from build123d import *

# Parameters (mm, degrees)
SZKIC1_W                    = 300
SZKIC1_H                    = 200
DODANIE_WYCI_GNI_CIE1_DEPTH = 2
WYTNIJ_WYCI_GNI_CIE1_REACH  = 182.289
SZKIC2_R                    = 1.5
WYTNIJ_WYCI_GNI_CIE2_DEPTH  = 2


with BuildPart() as part:
    # Szkic1 → Dodanie-wyciągnięcie1 (new body)
    with BuildSketch(Plane(origin=(0, 0, 0), x_dir=(1, 0, 0), z_dir=(0, 1, 0))):
        Rectangle(SZKIC1_W, SZKIC1_H)
    extrude(amount=-DODANIE_WYCI_GNI_CIE1_DEPTH)

    # Szkic2 → Wytnij-wyciągnięcie1 (cut, up to next)
    with BuildSketch(Plane(origin=(0, 0, 0), x_dir=(1, 0, 0), z_dir=(0, 1, 0)), mode=Mode.PRIVATE) as wytnij_wyci_gni_cie1_sk1:
        with Locations(Location((0, -86, 0), (0, 0, 270))):
            Circle(SZKIC2_R)
    wytnij_wyci_gni_cie1_tool1 = extrude(wytnij_wyci_gni_cie1_sk1.sketch, amount=-WYTNIJ_WYCI_GNI_CIE1_REACH, mode=Mode.PRIVATE) & part.part
    # Szkic2 → Wytnij-wyciągnięcie1 (cut, up to next)
    with BuildSketch(Plane(origin=(0, 0, 0), x_dir=(1, 0, 0), z_dir=(0, 1, 0)), mode=Mode.PRIVATE) as wytnij_wyci_gni_cie1_sk2:
        with Locations(Location((-7, -93, 0), (0, 0, 270))):
            Circle(SZKIC2_R)
    wytnij_wyci_gni_cie1_tool2 = extrude(wytnij_wyci_gni_cie1_sk2.sketch, amount=-WYTNIJ_WYCI_GNI_CIE1_REACH, mode=Mode.PRIVATE) & part.part
    # Szkic2 → Wytnij-wyciągnięcie1 (cut, up to next)
    with BuildSketch(Plane(origin=(0, 0, 0), x_dir=(1, 0, 0), z_dir=(0, 1, 0)), mode=Mode.PRIVATE) as wytnij_wyci_gni_cie1_sk3:
        with Locations(Location((7, -93, 0), (0, 0, 270))):
            Circle(SZKIC2_R)
    wytnij_wyci_gni_cie1_tool3 = extrude(wytnij_wyci_gni_cie1_sk3.sketch, amount=-WYTNIJ_WYCI_GNI_CIE1_REACH, mode=Mode.PRIVATE) & part.part
    # Szkic2 → Wytnij-wyciągnięcie1 (cut, up to next)
    with BuildSketch(Plane(origin=(0, 0, 0), x_dir=(1, 0, 0), z_dir=(0, 1, 0)), mode=Mode.PRIVATE) as wytnij_wyci_gni_cie1_sk4:
        with Locations(Location((-123, -86, 0), (0, 0, 270))):
            Circle(SZKIC2_R)
    wytnij_wyci_gni_cie1_tool4 = extrude(wytnij_wyci_gni_cie1_sk4.sketch, amount=-WYTNIJ_WYCI_GNI_CIE1_REACH, mode=Mode.PRIVATE) & part.part
    # Szkic2 → Wytnij-wyciągnięcie1 (cut, up to next)
    with BuildSketch(Plane(origin=(0, 0, 0), x_dir=(1, 0, 0), z_dir=(0, 1, 0)), mode=Mode.PRIVATE) as wytnij_wyci_gni_cie1_sk5:
        with Locations(Location((-130, -93, 0), (0, 0, 270))):
            Circle(SZKIC2_R)
    wytnij_wyci_gni_cie1_tool5 = extrude(wytnij_wyci_gni_cie1_sk5.sketch, amount=-WYTNIJ_WYCI_GNI_CIE1_REACH, mode=Mode.PRIVATE) & part.part
    # Szkic2 → Wytnij-wyciągnięcie1 (cut, up to next)
    with BuildSketch(Plane(origin=(0, 0, 0), x_dir=(1, 0, 0), z_dir=(0, 1, 0)), mode=Mode.PRIVATE) as wytnij_wyci_gni_cie1_sk6:
        with Locations(Location((-116, -93, 0), (0, 0, 270))):
            Circle(SZKIC2_R)
    wytnij_wyci_gni_cie1_tool6 = extrude(wytnij_wyci_gni_cie1_sk6.sketch, amount=-WYTNIJ_WYCI_GNI_CIE1_REACH, mode=Mode.PRIVATE) & part.part
    # Szkic2 → Wytnij-wyciągnięcie1 (cut, up to next)
    with BuildSketch(Plane(origin=(0, 0, 0), x_dir=(1, 0, 0), z_dir=(0, 1, 0)), mode=Mode.PRIVATE) as wytnij_wyci_gni_cie1_sk7:
        with Locations(Location((130, -93, 0), (0, 0, 270))):
            Circle(SZKIC2_R)
    wytnij_wyci_gni_cie1_tool7 = extrude(wytnij_wyci_gni_cie1_sk7.sketch, amount=-WYTNIJ_WYCI_GNI_CIE1_REACH, mode=Mode.PRIVATE) & part.part
    # Szkic2 → Wytnij-wyciągnięcie1 (cut, up to next)
    with BuildSketch(Plane(origin=(0, 0, 0), x_dir=(1, 0, 0), z_dir=(0, 1, 0)), mode=Mode.PRIVATE) as wytnij_wyci_gni_cie1_sk8:
        with Locations(Location((123, -86, 0), (0, 0, 270))):
            Circle(SZKIC2_R)
    wytnij_wyci_gni_cie1_tool8 = extrude(wytnij_wyci_gni_cie1_sk8.sketch, amount=-WYTNIJ_WYCI_GNI_CIE1_REACH, mode=Mode.PRIVATE) & part.part
    # Szkic2 → Wytnij-wyciągnięcie1 (cut, up to next)
    with BuildSketch(Plane(origin=(0, 0, 0), x_dir=(1, 0, 0), z_dir=(0, 1, 0)), mode=Mode.PRIVATE) as wytnij_wyci_gni_cie1_sk9:
        with Locations(Location((116, -93, 0), (0, 0, 270))):
            Circle(SZKIC2_R)
    wytnij_wyci_gni_cie1_tool9 = extrude(wytnij_wyci_gni_cie1_sk9.sketch, amount=-WYTNIJ_WYCI_GNI_CIE1_REACH, mode=Mode.PRIVATE) & part.part
    # Szkic2 → Wytnij-wyciągnięcie1 (cut, up to next)
    with BuildSketch(Plane(origin=(0, 0, 0), x_dir=(1, 0, 0), z_dir=(0, 1, 0)), mode=Mode.PRIVATE) as wytnij_wyci_gni_cie1_sk10:
        with Locations(Location((0, 86, 0), (0, 0, 270))):
            Circle(SZKIC2_R)
    wytnij_wyci_gni_cie1_tool10 = extrude(wytnij_wyci_gni_cie1_sk10.sketch, amount=-WYTNIJ_WYCI_GNI_CIE1_REACH, mode=Mode.PRIVATE) & part.part
    # Szkic2 → Wytnij-wyciągnięcie1 (cut, up to next)
    with BuildSketch(Plane(origin=(0, 0, 0), x_dir=(1, 0, 0), z_dir=(0, 1, 0)), mode=Mode.PRIVATE) as wytnij_wyci_gni_cie1_sk11:
        with Locations(Location((7, 93, 0), (0, 0, 270))):
            Circle(SZKIC2_R)
    wytnij_wyci_gni_cie1_tool11 = extrude(wytnij_wyci_gni_cie1_sk11.sketch, amount=-WYTNIJ_WYCI_GNI_CIE1_REACH, mode=Mode.PRIVATE) & part.part
    # Szkic2 → Wytnij-wyciągnięcie1 (cut, up to next)
    with BuildSketch(Plane(origin=(0, 0, 0), x_dir=(1, 0, 0), z_dir=(0, 1, 0)), mode=Mode.PRIVATE) as wytnij_wyci_gni_cie1_sk12:
        with Locations(Location((-7, 93, 0), (0, 0, 270))):
            Circle(SZKIC2_R)
    wytnij_wyci_gni_cie1_tool12 = extrude(wytnij_wyci_gni_cie1_sk12.sketch, amount=-WYTNIJ_WYCI_GNI_CIE1_REACH, mode=Mode.PRIVATE) & part.part
    # Szkic2 → Wytnij-wyciągnięcie1 (cut, up to next)
    with BuildSketch(Plane(origin=(0, 0, 0), x_dir=(1, 0, 0), z_dir=(0, 1, 0)), mode=Mode.PRIVATE) as wytnij_wyci_gni_cie1_sk13:
        with Locations(Location((130, 93, 0), (0, 0, 270))):
            Circle(SZKIC2_R)
    wytnij_wyci_gni_cie1_tool13 = extrude(wytnij_wyci_gni_cie1_sk13.sketch, amount=-WYTNIJ_WYCI_GNI_CIE1_REACH, mode=Mode.PRIVATE) & part.part
    # Szkic2 → Wytnij-wyciągnięcie1 (cut, up to next)
    with BuildSketch(Plane(origin=(0, 0, 0), x_dir=(1, 0, 0), z_dir=(0, 1, 0)), mode=Mode.PRIVATE) as wytnij_wyci_gni_cie1_sk14:
        with Locations(Location((123, 86, 0), (0, 0, 270))):
            Circle(SZKIC2_R)
    wytnij_wyci_gni_cie1_tool14 = extrude(wytnij_wyci_gni_cie1_sk14.sketch, amount=-WYTNIJ_WYCI_GNI_CIE1_REACH, mode=Mode.PRIVATE) & part.part
    # Szkic2 → Wytnij-wyciągnięcie1 (cut, up to next)
    with BuildSketch(Plane(origin=(0, 0, 0), x_dir=(1, 0, 0), z_dir=(0, 1, 0)), mode=Mode.PRIVATE) as wytnij_wyci_gni_cie1_sk15:
        with Locations(Location((116, 93, 0), (0, 0, 270))):
            Circle(SZKIC2_R)
    wytnij_wyci_gni_cie1_tool15 = extrude(wytnij_wyci_gni_cie1_sk15.sketch, amount=-WYTNIJ_WYCI_GNI_CIE1_REACH, mode=Mode.PRIVATE) & part.part
    # Szkic2 → Wytnij-wyciągnięcie1 (cut, up to next)
    with BuildSketch(Plane(origin=(0, 0, 0), x_dir=(1, 0, 0), z_dir=(0, 1, 0)), mode=Mode.PRIVATE) as wytnij_wyci_gni_cie1_sk16:
        with Locations(Location((-116, 93, 0), (0, 0, 270))):
            Circle(SZKIC2_R)
    wytnij_wyci_gni_cie1_tool16 = extrude(wytnij_wyci_gni_cie1_sk16.sketch, amount=-WYTNIJ_WYCI_GNI_CIE1_REACH, mode=Mode.PRIVATE) & part.part
    # Szkic2 → Wytnij-wyciągnięcie1 (cut, up to next)
    with BuildSketch(Plane(origin=(0, 0, 0), x_dir=(1, 0, 0), z_dir=(0, 1, 0)), mode=Mode.PRIVATE) as wytnij_wyci_gni_cie1_sk17:
        with Locations(Location((-123, 86, 0), (0, 0, 270))):
            Circle(SZKIC2_R)
    wytnij_wyci_gni_cie1_tool17 = extrude(wytnij_wyci_gni_cie1_sk17.sketch, amount=-WYTNIJ_WYCI_GNI_CIE1_REACH, mode=Mode.PRIVATE) & part.part
    # Szkic2 → Wytnij-wyciągnięcie1 (cut, up to next)
    with BuildSketch(Plane(origin=(0, 0, 0), x_dir=(1, 0, 0), z_dir=(0, 1, 0)), mode=Mode.PRIVATE) as wytnij_wyci_gni_cie1_sk18:
        with Locations(Location((-130, 93, 0), (0, 0, 270))):
            Circle(SZKIC2_R)
    wytnij_wyci_gni_cie1_tool18 = extrude(wytnij_wyci_gni_cie1_sk18.sketch, amount=-WYTNIJ_WYCI_GNI_CIE1_REACH, mode=Mode.PRIVATE) & part.part
    add(wytnij_wyci_gni_cie1_tool1.solids().sort_by_distance((0, 0, 86))[0], mode=Mode.SUBTRACT)
    add(wytnij_wyci_gni_cie1_tool2.solids().sort_by_distance((-7, 0, 93))[0], mode=Mode.SUBTRACT)
    add(wytnij_wyci_gni_cie1_tool3.solids().sort_by_distance((7, 0, 93))[0], mode=Mode.SUBTRACT)
    add(wytnij_wyci_gni_cie1_tool4.solids().sort_by_distance((-123, 0, 86))[0], mode=Mode.SUBTRACT)
    add(wytnij_wyci_gni_cie1_tool5.solids().sort_by_distance((-130, 0, 93))[0], mode=Mode.SUBTRACT)
    add(wytnij_wyci_gni_cie1_tool6.solids().sort_by_distance((-116, 0, 93))[0], mode=Mode.SUBTRACT)
    add(wytnij_wyci_gni_cie1_tool7.solids().sort_by_distance((130, 0, 93))[0], mode=Mode.SUBTRACT)
    add(wytnij_wyci_gni_cie1_tool8.solids().sort_by_distance((123, 0, 86))[0], mode=Mode.SUBTRACT)
    add(wytnij_wyci_gni_cie1_tool9.solids().sort_by_distance((116, 0, 93))[0], mode=Mode.SUBTRACT)
    add(wytnij_wyci_gni_cie1_tool10.solids().sort_by_distance((0, 0, -86))[0], mode=Mode.SUBTRACT)
    add(wytnij_wyci_gni_cie1_tool11.solids().sort_by_distance((7, 0, -93))[0], mode=Mode.SUBTRACT)
    add(wytnij_wyci_gni_cie1_tool12.solids().sort_by_distance((-7, 0, -93))[0], mode=Mode.SUBTRACT)
    add(wytnij_wyci_gni_cie1_tool13.solids().sort_by_distance((130, 0, -93))[0], mode=Mode.SUBTRACT)
    add(wytnij_wyci_gni_cie1_tool14.solids().sort_by_distance((123, 0, -86))[0], mode=Mode.SUBTRACT)
    add(wytnij_wyci_gni_cie1_tool15.solids().sort_by_distance((116, 0, -93))[0], mode=Mode.SUBTRACT)
    add(wytnij_wyci_gni_cie1_tool16.solids().sort_by_distance((-116, 0, -93))[0], mode=Mode.SUBTRACT)
    add(wytnij_wyci_gni_cie1_tool17.solids().sort_by_distance((-123, 0, -86))[0], mode=Mode.SUBTRACT)
    add(wytnij_wyci_gni_cie1_tool18.solids().sort_by_distance((-130, 0, -93))[0], mode=Mode.SUBTRACT)

    # Szkic3 → Wytnij-wyciągnięcie2 (cut)
    with BuildSketch(Plane.XZ.offset(2)):
        Polygon((-103, -100), (-83, -70), (-40, -70), (-20, -100), align=None)
        Polygon((103, -100), (83, -70), (40, -70), (20, -100), align=None)
        Polygon((103, 100), (20, 100), (40, 70), (83, 70), align=None)
        Polygon((-103, 100), (-83, 70), (-40, 70), (-20, 100), align=None)
    extrude(amount=-WYTNIJ_WYCI_GNI_CIE2_DEPTH, mode=Mode.SUBTRACT)


solid = part.part
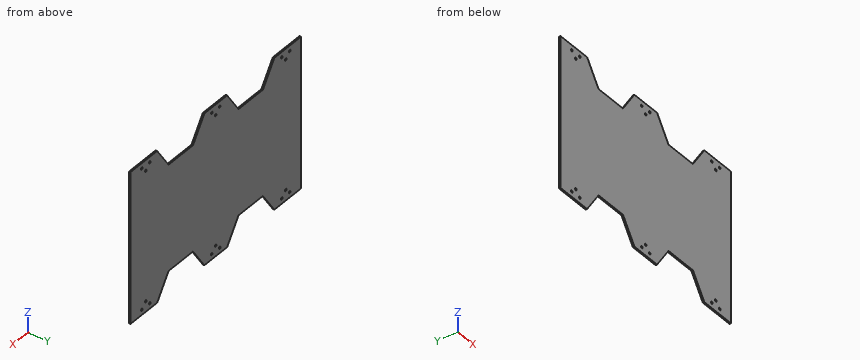
For this review, take the finished solid that the model builds, in its own axes (mm). Coordinates: 2 decimals unless noted, no trailing zeros. Write each loop counter-clockwise with the first axis right and the second up, starting at its lowest first coordinate (ties: lowest second). Pieces come first, ordered by that corner, then holes. Notation, with made-up numbers: (86, 86) -> (97, 86) arc R11 cw to (97, 93) -> close; hole circle Ø2 at (-8.75, 5.5). An arc over 180 degrees is marked (long way). Write each question's results on one line, items separated by ' | '. Start each with the question number.
1) Insertion check: pin 1 (1 mm diameter, centred on x = -51, y = -1, fed in from -Z). The pin has a flat end and moves straight along its axis. Give the tip position at first contact, or say it passes through.
2) Wall thickness on L1, parallel to Z at x = 130, y = -1.25; L2, parallel to X at y = -1.3, z = 86; L3, parallel to X at y = -1.15, z = 90: over which ranges is each line inside the solid? List them lowest first. Write a range as [from, to].
3) Consider section B-B (x = 71). Write out the cut boundary in (y, z), plus the area to 3 significant figures.
4) Consider section C-C (x = 28.5). Write out the cut boundary in (y, z).
5) Consider section A-A (y = -0.95). Give the number of separate pieces and of enclosed holes in the cut face, plus the area to 3 significant figures.
Geometry says:
1) pin 1: z = -70
2) L1: [-100, -94.5], [-91.5, 91.5], [94.5, 100] | L2: [-150, -124.5], [-121.5, -93.67], [-29.33, -1.5], [1.5, 29.33], [93.67, 121.5], [124.5, 150] | L3: [-150, -96.33], [-26.67, 26.67], [96.33, 150]
3) outline: (-2, -70) -> (0, -70) -> (0, 70) -> (-2, 70) -> close | area: 280 mm^2
4) outline: (-2, -87.25) -> (0, -87.25) -> (0, 87.25) -> (-2, 87.25) -> close
5) separate pieces: 1 | enclosed holes: 18 | area: 52,300 mm^2
